Could you check a few things on this model? Use its own coordinates, in mm. A direction names the side the tool comes from. Coordinates: 2 decimals unless noted, no trailing zeros. Order: outer loops, then holes, each group sorted by start corner. A loop starts at its lowest first (then second) coordinate and runs counter-clockwise, first axis right, second up. Notation, with made-up numbers: (61, 7) - (65, 7) arc R16 cw to (65, 21) - close; hole circle Ø10 at (49.25, -12). An arc over 180 degrees is marked (long way). Answer as CSV lines item,"result". Start each with the question number.
1. I want a section at D-D, the plane z = 0. Count the separate pieces of the cut face and the enclosed holes in it, and give its area (3 significant figures).
2. Thinking about a two-plate mould opening in Z: for faces 1 (the face through (-13.57, -0.07, -0.65)), 2 (the face through (5.81, 28.727, 0.358)), 3 (the face through (-10, 18, 0)), which applies, released by +Z, released by -Z, zero draft, split by the parting line, or undercut?
3. I want a section at C-C, the plane x = 3. List the corners of the cut face in (y, z) for me, and give its area (3 significant figures).
4. I want a section at A-A, the plane x = -16.5. List the corners of the cut face in (y, z) for me.
5. I want a section at B-B, the plane y = 26. List the corners of the cut face in (x, z) for me, and give its area (4 significant figures).
6. I need wall thicknesses on probe 1 along X at (y, z) = (0, 0); probe 2 along X at (y, z) = (23.5, 6.75); probe 3 along Y at (x, z) = (3, 0.75). Which ranges of each line are inside material? Lowest first, please.
7. For faces 4 (the face through (-5.15, 16.91, -0.14)), 5 (the face through (-19, 5, 2)), 6 (the face through (10, 19, 0)), 7 (the face through (-1.5, 11, 0)), 8 (the face through (-6, 32, 0)), which set-ups out of +Z, -Z, +X, -X, +Y, -Y let a thin tool reach every point of the face, with its end or its side?
8. For pin 1 (11 mm diameter, centred on y = 29, z = 4.5, fed in from -X); pin 2 (3 mm diameter, centred on y = 19.5, z = 2.5, fed in from +X); pin 3 (6.5 mm diameter, centred on x = 17.5, z = -4, fed in from +Y), each with a flat end and sliding along its axis, tell me the tip position at first contact or that it passes through.
Autodesk Inventor part; units mm, degrees
ref_plane "YZ Plane" through (0, 0, 0) normal (1, 0, 0) x (0, 1, 0)
ref_plane "XZ Plane" through (0, 0, 0) normal (0, 1, 0) x (-1, 0, 0)
ref_plane "XY Plane" through (0, 0, 0) normal (0, 0, 1) x (1, 0, 0)
sketch "Sketch1" plane through (0, 0, 0) normal (0, 0, 1) x (1, 0, 0)
  line L0 (-23, 5) -> (23, 5)
  line L1 (23, 5) -> (23, -5)
  line L2 (23, -5) -> (-23, -5)
  line L3 (-23, -5) -> (-23, 5)
  line L4 (-10, 32) -> (10, 32)
  line L5 (10, 32) -> (10, 5)
  line L6 (10, 5) -> (-10, 5)
  line L7 (-10, 5) -> (-10, 32)
  circle A0 centre (0, 17) radius 5.15
  line L8 (-1.5, 32) -> (1.5, 32)
  line L9 (1.5, 32) -> (1.5, 9)
  line L10 (1.5, 9) -> (-1.5, 9)
  line L11 (-1.5, 9) -> (-1.5, 32)
  point P0 (0, 0)
  point P1 (-23, 0)
  point P2 (0, 5)
  point P3 (0, 32)
  point P4 (0, 32)
  point P5 (-1.5, 12.0733)
  point P6 (-1.5, 21.9267)
  point P7 (-1.5, 32)
  point P8 (-10, 5)
  point P9 (10, 5)
  point P10 (1.5, 32)
  point P11 (1.5, 21.9267)
  point P12 (1.5, 12.0733)
  dimension "d0" = 10
  dimension "d1" = 20
  dimension "d2" = 10.3
  dimension "d3" = 12
  dimension "d4" = 15
  dimension "d5" = 3
  dimension "d6" = 8
  dimension "d7" = 13
extrude "Extrusion1" add sketch "Sketch1" along normal mid plane 20 contours L0 L1 L2 L3 | L7 L4 L11 A0 L10 L9 L5 L0
sketch "Sketch2" plane through (10, 5, 10) normal (0, 1, 0) x (1, 0, 0)
  line L0 (0, 20) -> (13, 20)
  line L1 (-33, 20) -> (-20, 20)
  line L2 (-33, 20) -> (-33, 0)
  line L3 (13, 20) -> (13, 0)
  point P0 (-10, 10)
  point P1 (-26.5, 10)
  point P2 (6.5, 10)
  point P3 (6.5, 20)
  point P4 (-26.5, 20)
  point P5 (-33, 10)
  point P6 (13, 10)
hole "Hole1" at (-16.5, 5, 0) at (16.5, 5, 0) direction (0, -1, 0) diameter 6 end through all
sketch "Sketch3" plane through (10, 5, 10) normal (1, 0, 0) x (0, 0, -1)
  line L0 (20, 27) -> (0, 27)
  circle A0 centre (10, 21) radius 2.75
  line L1 (20, 27) -> (0, 27)
  line L2 (0, 27) -> (8, 27)
  line L3 (8, 27) -> (8, 0)
  line L4 (8, 0) -> (0, 0)
  line L5 (0, 0) -> (0, 27)
  line L6 (20, 0) -> (0, 0)
  line L7 (12, 27) -> (20, 27)
  line L8 (20, 27) -> (20, 0)
  line L9 (20, 0) -> (12, 0)
  line L10 (12, 0) -> (12, 27)
  line L11 (20, 27) -> (20, 0)
  point P0 (10, -5)
  point P1 (10, 27)
  point P2 (12, 0)
  dimension "d17" = 6
  dimension "d18" = 5.5
  dimension "d19" = 8
  dimension "d21" = 8
extrude "Extrusion2" cut sketch "Sketch3" against normal through all contours L10 A0 L3 | A0 L10 | L3 A0
equation "\"d21\" = d19"
properties part number "0008-10-019 Suport Axa Y"
Solved:
1,separate pieces,"5"
1,enclosed holes,"0"
1,area,"665 mm2"
2,face 1,"undercut"
2,face 2,"undercut"
2,face 3,"zero draft"
3,outline,"(-5, -10) - (12.81, -10) - (12.81, 10) - (-5, 10) - close; (21.19, -10) - (32, -10) - (32, 10) - (21.19, 10) - close; hole circle Ø5.5 at (26, 0)"
3,area,"549 mm2"
4,outline,"(-5, -10) - (5, -10) - (5, -3) - (-5, -3) - close; (-5, 3) - (5, 3) - (5, 10) - (-5, 10) - close"
5,outline,"(-10, -10) - (-1.5, -10) - (-1.5, -2.75) - (-10, -2.75) - close; (-10, 2.75) - (-1.5, 2.75) - (-1.5, 10) - (-10, 10) - close; (1.5, -10) - (10, -10) - (10, -2.75) - (1.5, -2.75) - close; (1.5, 2.75) - (10, 2.75) - (10, 10) - (1.5, 10) - close"
5,area,"246.5 mm2"
6,probe 1,"x = -23 to -19.5, -13.5 to 13.5, 19.5 to 23"
6,probe 2,"x = -10 to -1.5, 1.5 to 10"
6,probe 3,"y = -5 to 12.81, 21.19 to 23.35, 28.65 to 32"
7,face 4,"+Z, -Z"
7,face 5,"+Z, -Z, -X, +Y"
7,face 6,"+Z, -Z, +X, +Y"
7,face 7,"+Z, -Z, +Y"
7,face 8,"+Z, -Z, +X, -X, +Y"
8,pin 1,"stops at x = -10"
8,pin 2,"stops at x = 10"
8,pin 3,"stops at y = 5"
